from build123d import *

# Parameters (mm, degrees)
F0_W     = 63
F0_H     = 70
F1_DEPTH = 12
F2_R     = 19.25
F3_DEPTH = 25
F4_R     = 4.25
F5_DEPTH = 63.001
F6_SIZE  = 1


with BuildPart() as f1:
    # F0 (on Front) → F1 (new body)
    with BuildSketch(Plane.XZ):
        with Locations((31.5, 35)):
            Rectangle(F0_W, F0_H)
    extrude(amount=F1_DEPTH)

    # F2 (on face) → F3 (cut)
    with BuildSketch(Plane.XZ.offset(12)):
        with Locations((31.5, 35)):
            Circle(F2_R)
    extrude(amount=-F3_DEPTH, mode=Mode.SUBTRACT)

    # F4 (on face) → F5 (cut, through all)
    with BuildSketch(Plane(origin=(0, 0, 0), x_dir=(0, -1, 0), z_dir=(-1, 0, 0))):
        with Locations((6, 61.5)):
            Circle(F4_R)
        with Locations((5.807274, 8.50035)):
            Circle(F4_R)
    extrude(amount=-F5_DEPTH, mode=Mode.SUBTRACT)

    # F6
    f6_edges = [f1.edges().sort_by_distance(p)[0] for p in [
        (63, -6, 70),
        (63, -6, 0),
        (0, -6, 0),
        (0, -6, 70),
    ]]
    chamfer(f6_edges, length=F6_SIZE)


solid = f1.part
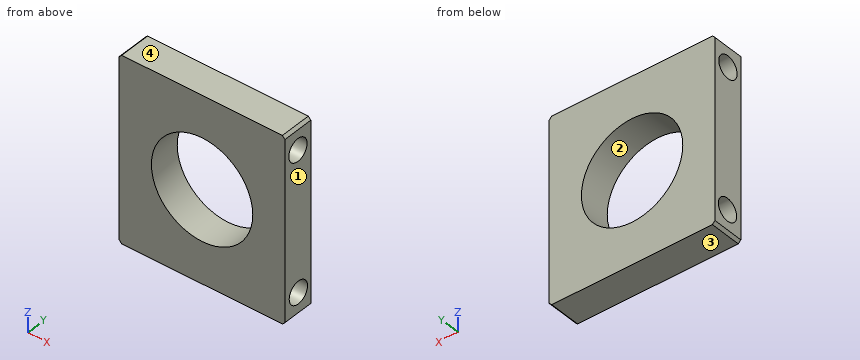
Source: CAD feature listing. Evaluate the final solid. Frame: model axes, mm. Face numbers are marked on the shaded views. Give positions to 0.01 mm unless a question says otherwise; leave off trailing zeros. Write each loop counter-clockwise with the first axis right and the second up, starting at its lowest first coordinate (ties: lowest second). Pieces come first, ordered by that corner, then holes. Notation, with made-up numbers: M -10,-36 L -5,-36 A31 cw -5,-12 Z; hole C -1.5,-0.75 d3. An arc over 180 degrees is marked long. Return JSON: item names as keys, results as strings. Group by question number.
1) Material intervals for line 1 along Z through (x, y) = (7.5, -4.5); line 2 along Z through (x, y) = (22.5, -5.5); line 3 along Z through (x, y) = (31.5, -4.5), sorted ascending. Write a range as [from, to].
2) Cut plane C-C, the plane x = 31.5. Output: boundary loops of the cut face in (y, z).
3) Pull-direction query (Z, two-part tool) for the marked faces 1, 2, 3 and 4; classes: pulls with the +Z half, pulls with the -Z half, needs draft (parallel to the pull), parting line crosses it, or undercut.
4) Cut plane A-A, the plane z = 61.5. Output: boundary loops of the cut face in (x, y).
5) Cut plane B-B, the plane y = -6. Output: boundary loops of the cut face in (x, z).
6) Cut plane D-D, the plane z = 35. Output: boundary loops of the cut face in (x, y).
Recorded:
{
 "1": {"line 1": "z = [0, 4.46], [12.54, 57.52], [65.48, 70]", "line 2": "z = [0, 4.26], [12.74, 17.98], [52.02, 57.28], [65.72, 70]", "line 3": "z = [0, 4.46], [12.54, 15.75], [54.25, 57.52], [65.48, 70]"},
 "2": {"outline": "M -12,0 L 0,0 L 0,15.75 L -12,15.75 Z; M -12,54.25 L 0,54.25 L 0,70 L -12,70 Z; hole C -6,61.5 d8.5; hole C -5.81,8.5 d8.5"},
 "3": {"face 1": "needs draft", "face 2": "undercut", "face 3": "pulls with the -Z half", "face 4": "pulls with the +Z half"},
 "4": {"outline": "M 0,-12 L 63,-12 L 63,-10.25 L 0,-10.25 Z; M 0,-1.75 L 63,-1.75 L 63,0 L 0,0 Z"},
 "5": {"outline": "M 0,1 L 1,0 L 62,0 L 63,1 L 63,4.25 L 0,4.25 Z; M 0,12.75 L 63,12.75 L 63,57.25 L 0,57.25 Z; M 0,65.75 L 63,65.75 L 63,69 L 62,70 L 1,70 L 0,69 Z; hole C 31.5,35 d38.5"},
 "6": {"outline": "M 0,-12 L 12.25,-12 L 12.25,0 L 0,0 Z; M 50.75,-12 L 63,-12 L 63,0 L 50.75,0 Z"}
}
